Part model, mm, in its own coordinate system. Give positions to 0.01 mm unless a question says otherwise; leave off trailing zeros. Loops run counter-clockwise (first coordinate to the right, second up) from the corner with the lowest first, then second, coordinate; pieces in that order, holes last. Notation, with made-up numbers: (-31.5, 82.25) -> (-5.5, 82.25) arc R18 ccw to (-5.5, 113.25) -> close; hole circle Ø3 at (46, -21). An arc over 180 degrees is marked (long way). Write item = value, one per line.
from build123d import *

# Parameters (mm, degrees)
SKETCH1_W           = 30
SKETCH1_H           = 30
SKETCH1_R           = 1.55
BOSS_EXTRUDE1_DEPTH = 20
SKETCH3_R           = 2
CUT_EXTRUDE1_DEPTH  = 10


with BuildPart() as part:
    # Sketch1 → Boss-Extrude1 (new body)
    with BuildSketch(Plane.XY):
        Rectangle(SKETCH1_W, SKETCH1_H)
        with Locations((-10.960155108, 10.960155108)):
            Circle(SKETCH1_R, mode=Mode.SUBTRACT)
        with Locations((10.960155108, 10.960155108)):
            Circle(SKETCH1_R, mode=Mode.SUBTRACT)
        with Locations((10.960155108, -10.960155108)):
            Circle(SKETCH1_R, mode=Mode.SUBTRACT)
        with Locations((-10.960155108, -10.960155108)):
            Circle(SKETCH1_R, mode=Mode.SUBTRACT)
    extrude(amount=BOSS_EXTRUDE1_DEPTH)

    # Sketch3 → Cut-Extrude1 (cut)
    with BuildSketch(Plane.XY.offset(20)):
        Circle(SKETCH3_R)
    extrude(amount=-CUT_EXTRUDE1_DEPTH, mode=Mode.SUBTRACT)


solid = part.part
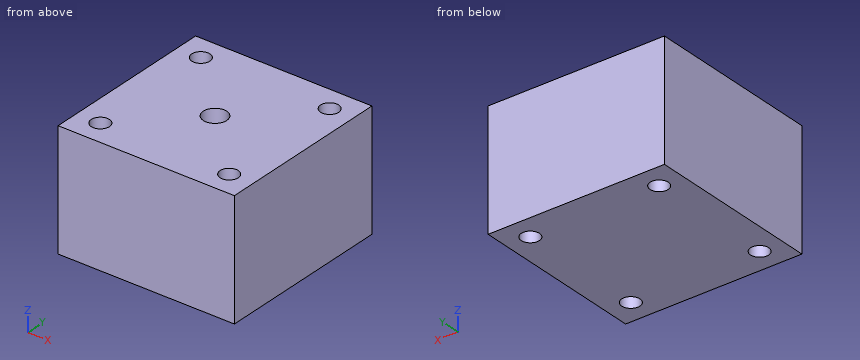
1) Drop flat-ended pins along their axis: P1, Ø2.5, axis at x = 10.96, y = -10.96, coming from the +Z side (3 decimals); P2, Ø3, axis at x = 0, y = 0, coming from the +Z side. Give the stop position or say it passes through.
Resolved:
P1 = through
P2 = 10
2) Slice it at A-A, the plane x = 10.25. List the corners of the cut face in (y, z), and give its area (3 significant figures).
Resolved:
outline = (-15, 0) -> (-12.34, 0) -> (-12.34, 20) -> (-15, 20) -> close; (-9.58, 0) -> (9.58, 0) -> (9.58, 20) -> (-9.58, 20) -> close; (12.34, 0) -> (15, 0) -> (15, 20) -> (12.34, 20) -> close
area = 490 mm²
3) Drill centre lines: line 1 along Y through (x, z) = (-11, 12.5); line 2 along Y through (x, z) = (0, 16.5); line 3 along X through (y, z) = (-11.75, 2.75). Where is each one in solid material? Low to high. Write a range as [from, to].
Resolved:
line_1 = [-15, -12.51], [-9.41, 9.41], [12.51, 15]
line_2 = [-15, -2], [2, 15]
line_3 = [-15, -12.29], [-9.63, 9.63], [12.29, 15]
4) Slice it at D-D, the plane x = 0. List the corners of the cut face in (y, z), and give its area (3 significant figures).
Resolved:
outline = (-15, 0) -> (15, 0) -> (15, 20) -> (2, 20) -> (2, 10) -> (-2, 10) -> (-2, 20) -> (-15, 20) -> close
area = 560 mm²
5) Slice it at C-C, the plane z = 15.5. List the corners of the cut face in (x, y).
Resolved:
outline = (-15, -15) -> (15, -15) -> (15, 15) -> (-15, 15) -> close; hole circle Ø3.1 at (-10.96, -10.96); hole circle Ø3.1 at (-10.96, 10.96); hole circle Ø4 at (0, 0); hole circle Ø3.1 at (10.96, -10.96); hole circle Ø3.1 at (10.96, 10.96)
